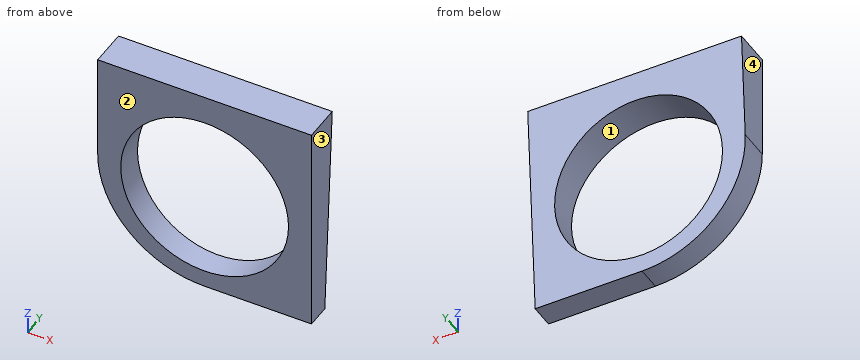
```python
from build123d import *

# Parameters (mm, degrees)
SKETCH1_R           = 17.5
BOSS_EXTRUDE1_DEPTH = 300
CUT_EXTRUDE1_DEPTH  = 150


with BuildPart() as part:
    # Sketch1 → Boss-Extrude1 (new body)
    with BuildSketch(Plane(origin=(0, 0, 0), x_dir=(1, 0, 0), z_dir=(0, 1, 0))):
        with BuildLine():
            Line((-22.3, -23.5), (22.3, -23.5))
            Line((22.3, -23.5), (22.3, 21.1))
            Line((22.3, 21.1), (0, 21.1))
            ThreePointArc((0, 21.1), (-15.76848122, 14.56848122), (-22.3, -1.2))
            Line((-22.3, -1.2), (-22.3, -23.5))
        make_face()
        Circle(SKETCH1_R, mode=Mode.SUBTRACT)
    extrude(amount=BOSS_EXTRUDE1_DEPTH)

    # Sketch2 → Cut-Extrude1 (cut, symmetric)
    with BuildSketch(Plane(origin=(0, 0, 0), x_dir=(0, 0, -1), z_dir=(1, 0, 0))):
        Polygon((-23.5, 7.8), (21.1, 5), (89.895743618, 5), (89.895743618, 331.939309381), (-23.5, 331.939309381), align=None)
    extrude(amount=CUT_EXTRUDE1_DEPTH, both=True, mode=Mode.SUBTRACT)


solid = part.part
```
Can you work these out from the model? Positions are in its coordinate system, mm. Face numbers are marked on the shaded views. Coordinates: 2 decimals unless noted, no trailing zeros. Loops run counter-clockwise (first coordinate to the right, second up) from the corner with the lowest first, then second, coordinate; pieces in that order, holes last. Notation, with made-up numbers: (-15, -3) -> (1, -3) arc R18 cw to (1, 12) -> close; hole circle Ø1 at (61, 49.5). An arc over 180 degrees is marked (long way). Answer as a JSON object with one key per item and string values.
1) Thinking about a two-plate mould opening in X: for the marked faces 1, 2, 3 and 4, which applies, pulls with the +X half, pulls with the -X half, needs draft (parallel to the pull), parting line crosses it, or undercut?
Results:
{"face 1": "undercut", "face 2": "needs draft", "face 3": "pulls with the +X half", "face 4": "pulls with the -X half"}
2) Imagine slicing it at A-A (x = -16.5). Please give me the cut outline in (y, z).
Results:
{"outline": "(0, -13.8) -> (5.46, -13.8) -> (5.96, -5.83) -> (0, -5.83) -> close; (0, 5.83) -> (6.69, 5.83) -> (7.8, 23.5) -> (0, 23.5) -> close"}
3) Imagine slicing it at B-B (y = 2.5). Please give me the cut outline in (x, z), then the cut area to 3 significant figures.
Results:
{"outline": "(-22.3, 1.2) arc R22.3 ccw to (0, -21.1) -> (22.3, -21.1) -> (22.3, 23.5) -> (-22.3, 23.5) -> close; hole circle Ø35 at (0, 0)", "area": "920 mm^2"}
4) For P1, Ø6, axis at x = 5, z = 13, coming from the +Y side; P2, Ø1.5, axis at x = -9, y = 4.5, coming from the -Z side, each with a flat end and sliding along its axis, tell me the tip position at first contact or that it passes through.
Results:
{"P1": "passes through", "P2": "stops at z = -19.52"}
5) If I drill on line 1 (Z direction, x = 0, y = 4.5); line 2 (X direction, y = 4.5, z = -12.5); line 3 (Z direction, x = -3, y = 4.75), over which ranges is the centre line in solid material (lowest first)?
Results:
{"line 1": "z = -21.1 to -17.5, 17.5 to 23.5", "line 2": "x = -17.6 to -12.25, 12.25 to 22.3", "line 3": "z = -20.9 to -17.24, 17.24 to 23.5"}
6) Imagine slicing it at C-C (z = 15). Please give me the cut outline in (x, y).
Results:
{"outline": "(-22.3, 0) -> (-9.01, 0) -> (-9.01, 7.27) -> (-22.3, 7.27) -> close; (9.01, 0) -> (22.3, 0) -> (22.3, 7.27) -> (9.01, 7.27) -> close"}
